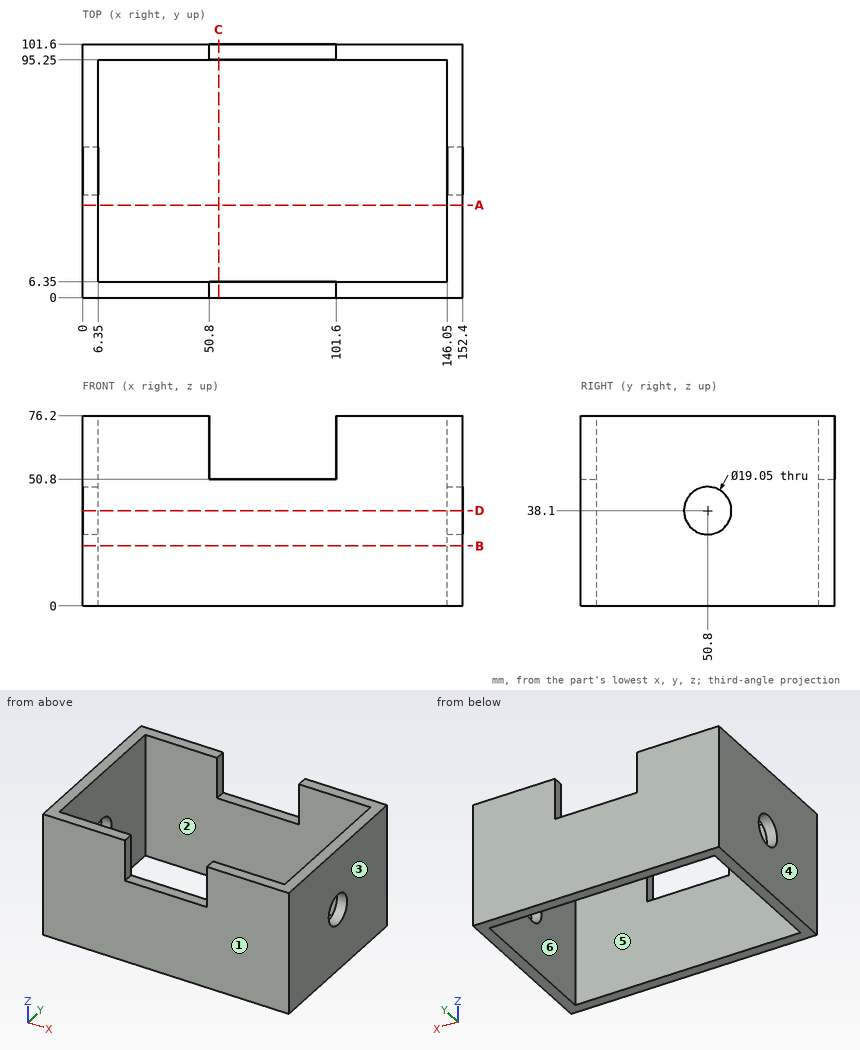
Here's the drawing with two shaded views (mm, measured from the low corner). I have some questions. A direction names the side the tool comes from. Round coordinates to 2 decimals unless told otherwise and drop trailing zeros. Order: outer loops, then holes, each group sorted by start corner. A loop starts at its lowest first (then second) coordinate and runs counter-clockwise, first axis right, second up. Notation, with made-up numbers: M 52,70 L 77,70 A23 cw 77,100 Z; hole C 77.25,18 d1. An arc over 180 degrees is marked long. Use CSV: the item, a comma, the result in double quotes.
1) I want a section at B-B (z = 24). List the corners of the cut face in (x, y) for me.
Taken from the geometry:
outline,"M 0,0 L 152.4,0 L 152.4,101.6 L 0,101.6 Z; hole M 6.35,6.35 L 146.05,6.35 L 146.05,95.25 L 6.35,95.25 Z"
2) On a 3-axis mill with a long thin cutter (end or side, diameter ignored), from which of +Z, -Z, +X, -X, +Y, -Y can I reach the whole of each face in a straight line? I mean the marked faces 1 and 2. Say none if no direction works.
Taken from the geometry:
face 1,"+Z, -Z, +X, -X, -Y"
face 2,"+Z, -Z"
3) I'm going to push flat-ended pins straight in: P1, Ø3, axis at x = 71, y = 98.5, coming from the +Z side; P2, Ø17, axis at y = 50.8, z = 38.1, coming from the +X side. Where does each tip first touch, or does it pass through?
Taken from the geometry:
P1,"z = 50.8"
P2,"through"
4) I need wall thicknesses on line 1 along Z through (x, y) = (149, 50); line 2 along Y through (x, z) = (33.5, 7); line 3 along X through (y, z) = (30.5, 8.5). Which ranges of each line are inside material? Lowest first, please. Write a range as [from, to].
Taken from the geometry:
line 1,"[0, 28.61], [47.59, 76.2]"
line 2,"[0, 6.35], [95.25, 101.6]"
line 3,"[0, 6.35], [146.05, 152.4]"
5) I want a section at C-C (x = 54.5). List the corners of the cut face in (y, z) for me, then the cut area to 3 significant figures.
Taken from the geometry:
outline,"M 0,0 L 6.35,0 L 6.35,50.8 L 0,50.8 Z; M 95.25,0 L 101.6,0 L 101.6,50.8 L 95.25,50.8 Z"
area,"645 mm^2"
6) I want a section at D-D (z = 38.1). List the corners of the cut face in (x, y) for me (3 decimals), then the cut area to 3 significant figures.
Taken from the geometry:
outline,"M 0,0 L 152.4,0 L 152.4,41.275 L 146.05,41.275 L 146.05,6.35 L 6.35,6.35 L 6.35,41.275 L 0,41.275 Z; M 0,60.325 L 6.35,60.325 L 6.35,95.25 L 146.05,95.25 L 146.05,60.325 L 152.4,60.325 L 152.4,101.6 L 0,101.6 Z"
area,"2,820 mm^2"
7) I want a section at A-A (y = 37). List the corners of the cut face in (x, z) for me, then the cut area to 3 significant figures.
Taken from the geometry:
outline,"M 0,0 L 6.35,0 L 6.35,76.2 L 0,76.2 Z; M 146.05,0 L 152.4,0 L 152.4,76.2 L 146.05,76.2 Z"
area,"968 mm^2"
8) If we mould it in two halves opening along X, with no side actions, what happens to the marked faces 3, 4, 5 and 6? For each: pulls with the +X half, pulls with the -X half, needs draft (parallel to the pull), parting line crosses it, or undercut.
Taken from the geometry:
face 3,"pulls with the +X half"
face 4,"pulls with the -X half"
face 5,"undercut"
face 6,"undercut"
